Here's how the part is built. I have some questions about the finished solid (model axes, mm). A direction names the side the tool comes from. Coordinates: 2 decimals unless noted, no trailing zeros. Write each loop counter-clockwise with the first axis right and the second up, starting at its lowest first coordinate (ties: lowest second). Pieces come first, ordered by that corner, then holes.
Item 1: I want a section at A-A (y = 28.5). Please give me the cut outline in (x, z), and give its area (3 significant figures).
Item 2: I'm going to push flat-ended pins straight in: P1, Ø4, axis at x = 14.5, z = -2.5, coming from the +Y side; P2, Ø3, axis at y = 26.5, z = 13.5, coming from the +X side; P3, Ø3, axis at y = 26.5, z = -15, coming from the -X side; P4, Ø0.8, axis at x = -20.5, y = 12.5, coming from the -Z side. Where does each tip first touch, or does it pass through?
Item 3: For faces 1 (the face through (-19.8, 27, 16.4)), 2 (the face through (0, 25.5, 0)), 3 (the face through (10.8, 27, -16.5)), 4 (the face through (-21, 6, 0)), which set-ups out of +Z, -Z, +X, -X, +Y, -Y let a thin tool reach every point of the face, with its end or its side?
Item 4: I want a section at D-D (y = -2). Please give me the cut outline in (x, z), and give its area (3 significant figures).
Item 5: Please list where these lines run through material, in increasing order: line 1 (X direction, y = 19, z = -6.5); line 2 (Y direction, x = -5.5, z = -7); line 3 (Y direction, x = 21.65, z = 0).
Item 6: I want a section at B-B (z = 0). Please give me the cut outline in (x, y), and give its area (3 significant figures).
Item 7: If we mould it in two halves opening along Z, with no side actions, what happens to faces 5 (the face through (-4.71, 24.43, -17.05)), 6 (the face through (-19.8, 27, -16.5)), 7 (the face through (-4, 29, 16))? For each: pulls with the +Z half, pulls with the -Z half, needs draft (parallel to the pull), parting line crosses it, or undercut.
Item 8: I want a section at C-C (x = 6.5). Please give me the cut outline in (y, z), and give its area (3 significant figures).
from build123d import *

# Parameters (mm, degrees)
BOSS_EXTRUDE1_DEPTH          = 45
SKETCH2_W                    = 42
SKETCH2_H                    = 41.882656114
CUT_EXTRUDE1_DEPTH           = 23
SKETCH3_W                    = 30.6
SKETCH3_H                    = 1.5
BOSS_EXTRUDE2_DEPTH          = 6.5
SKETCH4_W                    = 30.6
SKETCH4_H                    = 1.5
BOSS_EXTRUDE3_DEPTH          = 6.3
SKETCH5_W                    = 30.6
SKETCH5_H                    = 1.5
BOSS_EXTRUDE4_DEPTH          = 6.5
SKETCH6_W                    = 30.6
SKETCH6_H                    = 1.5
BOSS_EXTRUDE5_DEPTH          = 6.3
F_8_0_8_DIAMETER_HOLE1_D     = 8
F_8_0_8_DIAMETER_HOLE1_DEPTH = 1.5
F_8_0_8_DIAMETER_HOLE2_D     = 8
F_8_0_8_DIAMETER_HOLE2_DEPTH = 1.5
FILLET1_R                    = 1.5


with BuildPart() as part:
    # Sketch1 → Boss-Extrude1 (new body)
    with BuildSketch(Plane(origin=(-22.5, 0, 0), x_dir=(0, -1, 0), z_dir=(-1, 0, 0))):
        with BuildLine():
            Line((-25.5, -11), (0, -11))
            ThreePointArc((0, -11), (11, 0), (0, 11))
            Line((0, 11), (-25.5, 11))
            Line((-25.5, 11), (-25.5, -11))
        make_face()
    extrude(amount=-BOSS_EXTRUDE1_DEPTH)

    # Sketch2 → Cut-Extrude1 (cut, through all)
    with BuildSketch(Plane.XY.offset(11)):
        with Locations((0, 3.058671943)):
            Rectangle(SKETCH2_W, SKETCH2_H)
    extrude(amount=-CUT_EXTRUDE1_DEPTH, mode=Mode.SUBTRACT)

    # Sketch3 → Boss-Extrude2 (add)
    with BuildSketch(Plane(origin=(0, 0, -11), x_dir=(-1, 0, 0), z_dir=(0, 0, -1))):
        with Locations((4.5, 24.75)):
            Rectangle(SKETCH3_W, SKETCH3_H)
    extrude(amount=BOSS_EXTRUDE2_DEPTH)

    # Sketch4 → Boss-Extrude3 (add)
    with BuildSketch(Plane(origin=(0, 25.5, 0), x_dir=(-1, 0, 0), z_dir=(0, 1, 0))):
        with Locations((4.5, -16.75)):
            Rectangle(SKETCH4_W, SKETCH4_H)
    extrude(amount=BOSS_EXTRUDE3_DEPTH)

    # Sketch5 → Boss-Extrude4 (add)
    with BuildSketch(Plane.XY.offset(11)):
        with Locations((-4.5, 24.75)):
            Rectangle(SKETCH5_W, SKETCH5_H)
    extrude(amount=BOSS_EXTRUDE4_DEPTH)

    # Sketch6 → Boss-Extrude5 (add)
    with BuildSketch(Plane(origin=(0, 25.5, 0), x_dir=(-1, 0, 0), z_dir=(0, 1, 0))):
        with Locations((4.5, 16.75)):
            Rectangle(SKETCH6_W, SKETCH6_H)
    extrude(amount=BOSS_EXTRUDE5_DEPTH)

    # Ø8.0 (8) Diameter Hole1
    with Locations(Plane.ZY.offset(-21)):
        with Locations((0, 0)):
            Hole(F_8_0_8_DIAMETER_HOLE1_D / 2, depth=F_8_0_8_DIAMETER_HOLE1_DEPTH)

    # Ø8.0 (8) Diameter Hole2
    with Locations(Plane(origin=(-21, 0, 0), x_dir=(0, 0, -1), z_dir=(1, 0, 0))):
        with Locations((0, 0)):
            Hole(F_8_0_8_DIAMETER_HOLE2_D / 2, depth=F_8_0_8_DIAMETER_HOLE2_DEPTH)

    # Fillet1
    fillet1_edges = [part.edges().sort_by_distance(p)[0] for p in [
        (-4.5, 24, -17.5),
        (22.5, 25.5, 0),
        (-22.5, 25.5, 0),
        (-4.5, 24, 17.5),
    ]]
    fillet(fillet1_edges, radius=FILLET1_R)


solid = part.part
Answer:
1. outline: (-19.8, -17.5) - (10.8, -17.5) - (10.8, -16) - (-19.8, -16) - close; (-19.8, 16) - (10.8, 16) - (10.8, 17.5) - (-19.8, 17.5) - close
1. area: 91.8 mm2
2. P1: stops at y = 25.5
2. P2: stops at x = 10.8
2. P3: stops at x = -19.8
2. P4: passes through
3. face 1: +Z, -X, +Y, -Y
3. face 2: +X, -X, +Y
3. face 3: -Z, +X, +Y, -Y
3. face 4: +Z, -Z, -Y
4. outline: (-22.5, -10.82) - (-21, -10.82) - (-21, -3.46) - (-22.5, -3.46) - close; (-22.5, 3.46) - (-21, 3.46) - (-21, 10.82) - (-22.5, 10.82) - close; (21, -10.82) - (22.5, -10.82) - (22.5, -3.46) - (21, -3.46) - close; (21, 3.46) - (22.5, 3.46) - (22.5, 10.82) - (21, 10.82) - close
4. area: 44.1 mm2
5. line 1: x = -22.5 to -21, 21 to 22.5
5. line 2: y = 24 to 25.5
5. line 3: y = -11 to -4, 4 to 25.35
6. outline: (-22.5, -11) - (-21, -11) - (-21, -4) - (-22.5, -4) - close; (-22.5, 4) - (-21, 4) - (-21, 24) - (21, 24) - (21, 4) - (22.5, 4) - (22.5, 24) arc R1.5 ccw to (21, 25.5) - (-21, 25.5) arc R1.5 ccw to (-22.5, 24) - close; (21, -11) - (22.5, -11) - (22.5, -4) - (21, -4) - close
6. area: 148 mm2
7. face 5: pulls with the -Z half
7. face 6: needs draft
7. face 7: undercut
8. outline: (24, -16) arc R1.5 ccw to (25.5, -17.5) - (31.8, -17.5) - (31.8, -16) - (25.5, -16) - (25.5, 16) - (31.8, 16) - (31.8, 17.5) - (25.5, 17.5) arc R1.5 ccw to (24, 16) - close
8. area: 70.4 mm2
